Here's how the part is built. I have some questions about the finished solid (model axes, mm). A direction names the side the tool comes from. Give positions to 0.01 mm unless a question says otherwise; leave off trailing zeros. Loops run counter-clockwise (first coordinate to the right, second up) from the corner with the lowest first, then second, coordinate; pieces in that order, holes last. Notation, with made-up numbers: (58.25, 70.5) - (73.25, 70.5) arc R24 cw to (73.25, 83.5) - close; hole circle Ø4 at (-12, 83.5). An arc over 180 degrees is marked (long way). Use a Markdown table: item, result.
from build123d import *

# Parameters (mm, degrees)
SKETCH1_R           = 11.3
SKETCH1_R_2         = 4
SKETCH1_R_3         = 2
BOSS_EXTRUDE1_DEPTH = 2
FILLET1_R           = 10
SKETCH2_R           = 2.1
CUT_EXTRUDE1_DEPTH  = 182.73882359


with BuildPart() as part:
    # Sketch1 → Boss-Extrude1 (new body)
    with BuildSketch(Plane.XY):
        with BuildLine():
            ThreePointArc((0, 0), (12.5, -12.5), (25, 0))
            Line((25, 0), (25, 15))
            Line((25, 15), (17, 15))
            Line((17, 15), (17, 137.5))
            Line((17, 137.5), (25, 137.5))
            Line((25, 137.5), (25, 180))
            Line((25, 180), (0, 180))
            Line((0, 180), (0, 137.5))
            Line((0, 137.5), (8, 137.5))
            Line((8, 137.5), (8, 15))
            Line((8, 15), (0, 15))
            Line((0, 15), (0, 0))
        make_face()
        with Locations((12.5, 0)):
            Circle(SKETCH1_R, mode=Mode.SUBTRACT)
        with Locations((12.5, 150)):
            Circle(SKETCH1_R_2, mode=Mode.SUBTRACT)
        with Locations((18.156854249, 144.343145751)):
            Circle(SKETCH1_R_3, mode=Mode.SUBTRACT)
        with Locations((5.782485579, 143.282485579)):
            Circle(SKETCH1_R_3, mode=Mode.SUBTRACT)
        with Locations((19.217514421, 156.717514421)):
            Circle(SKETCH1_R_3, mode=Mode.SUBTRACT)
        with Locations((6.843145751, 155.656854249)):
            Circle(SKETCH1_R_3, mode=Mode.SUBTRACT)
    extrude(amount=BOSS_EXTRUDE1_DEPTH)

    # Fillet1
    # the kernel refuses this fillet: 10 mm, written as the material it takes off along each edge
    with BuildSketch(Plane(origin=(25, 15, -24.494897428), x_dir=(0, -1, 0), z_dir=(0, 0, 1)), Plane(origin=(0, 137.5, -24.494897428), x_dir=(0, 1, 0), z_dir=(0, 0, 1))) as fillet1_piece_1:
        with BuildLine():
            CenterArc((9.797958971, -10), FILLET1_R, 90, 78.463040967)
            Line((0, -8), (-0.195959179, -7.96))
            ThreePointArc((-0.195959179, -7.96), (-0.2, -4), (-0.2, 0))
            Line((-0.2, 0), (0, 0.2))
            Line((0, 0.2), (9.797958971, 0.2))
            Line((9.797958971, 0.2), (9.797958971, 0))
        make_face()
    extrude(amount=50.989794856, mode=Mode.SUBTRACT)
    with BuildSketch(Plane(origin=(0, 15, -24.494897428), x_dir=(1, 0, 0), z_dir=(0, 0, 1)), Plane(origin=(25, 137.5, -24.494897428), x_dir=(-1, 0, 0), z_dir=(0, 0, 1))) as fillet1_piece_2:
        with BuildLine():
            CenterArc((10, -9.797958971), FILLET1_R, 101.536959033, 78.463040967)
            Line((0, -9.797958971), (-0.2, -9.797958971))
            Line((-0.2, -9.797958971), (-0.2, 0))
            Line((-0.2, 0), (0, 0.2))
            ThreePointArc((0, 0.2), (4, 0.2), (7.96, 0.195959179))
            Line((7.96, 0.195959179), (8, 0))
        make_face()
    extrude(amount=50.989794856, mode=Mode.SUBTRACT)
    with BuildSketch(Plane(origin=(0, 180, -25), x_dir=(1, 0, 0), z_dir=(0, 0, 1)), Plane(origin=(25, 180, -25), x_dir=(0, -1, 0), z_dir=(0, 0, 1))) as fillet1_piece_3:
        with BuildLine():
            CenterArc((FILLET1_R, -FILLET1_R), FILLET1_R, 90, 90)
            Line((0, -FILLET1_R), (-FILLET1_R * 0.02, -FILLET1_R))
            Line((-FILLET1_R * 0.02, -FILLET1_R), (-FILLET1_R * 0.02, FILLET1_R * 0.02))
            Line((-FILLET1_R * 0.02, FILLET1_R * 0.02), (FILLET1_R, FILLET1_R * 0.02))
            Line((FILLET1_R, FILLET1_R * 0.02), (FILLET1_R, 0))
        make_face()
    extrude(amount=52, mode=Mode.SUBTRACT)

    # Sketch2 → Cut-Extrude1 (cut, through all)
    with BuildSketch(Plane(origin=(0, 0, 0), x_dir=(-1, 0, 0), z_dir=(0, 0, -1))):
        with Locations((-12.5, 120)):
            Circle(SKETCH2_R)
        with Locations((-12.5, 30)):
            Circle(SKETCH2_R)
        with Locations((-19.5, 170)):
            Circle(SKETCH2_R)
        with Locations(Location((-5.5, 170, 0), (0, 0, 180))):
            Circle(SKETCH2_R)
    extrude(amount=-CUT_EXTRUDE1_DEPTH, mode=Mode.SUBTRACT)


solid = part.part
(1) Suppose I cut it at A-A on y = 120. Write out the boundary of the cut face in (x, z), plus the area to 3 significant figures.
A:
| item | result |
|---|---|
| outline | (8, 0) - (10.4, 0) - (10.4, 2) - (8, 2) - close; (14.6, 0) - (17, 0) - (17, 2) - (14.6, 2) - close |
| area | 9.60 mm2 |
(2) We'd pull the mould along Y, two halves only. Please class faces 4 (the face through (22.15, 176.99, 0.99)), 5 (the face through (12.225, -12.497, 0.986)), 6 (the face through (1.21, 0.5, 0.99)): pulls with the +Y half, pulls with the -Y half, needs draft (parallel to the pull), parting line crosses it, or undercut.
A:
| item | result |
|---|---|
| face 4 | pulls with the +Y half |
| face 5 | pulls with the -Y half |
| face 6 | undercut |
(3) Suppose I cut it at C-C on y = 150. Write out the boundary of the cut face in (x, z), plus the area to 3 significant figures.
A:
| item | result |
|---|---|
| outline | (0, 0) - (8.5, 0) - (8.5, 2) - (0, 2) - close; (16.5, 0) - (25, 0) - (25, 2) - (16.5, 2) - close |
| area | 34.0 mm2 |
(4) Suppose I cut it at B-B on z = 1.45. Count the separate pieces of the cut face and the enclosed holes in it, plus the area to 3 significant figures.
A:
| item | result |
|---|---|
| separate pieces | 1 |
| enclosed holes | 10 |
| area | 2,110 mm2 |
(5) If I drill on line 1 (Y direction, x = 12.5, z = 1.15); line 2 (Y direction, x = 13.25, z = 0.4); line 3 (Y direction, x = 6.25, z = 0.9), over which ranges is the centre line in solid material (lowest first)?
A:
| item | result |
|---|---|
| line 1 | -12.5 to -11.3, 11.3 to 27.9, 32.1 to 117.9, 122.1 to 146, 154 to 180 |
| line 2 | -12.48 to -11.28, 11.28 to 28.04, 31.96 to 118.04, 121.96 to 146.07, 153.93 to 180 |
| line 3 | -10.83 to -9.41, 9.41 to 14.47, 138.03 to 141.34, 145.23 to 153.75, 157.57 to 168.04, 171.96 to 179.27 |
(6) Will these pins go through, and if not, where does the flat tip stop? pin 1 (1 mm diameter, centred on y = 59, z = 1.5, fed in from +X); pin 2 (0.6 mm diameter, centred on y = 90.5, z = 1, fed in from -X).
A:
| item | result |
|---|---|
| pin 1 | x = 17 |
| pin 2 | x = 8 |
(7) On a 3-axis mill with a long thin cutter (end or side, diameter ignored), from which of +Z, -Z, +X, -X, +Y, -Y can I reach the whole of each face in a straight line? I mean faces 1 (the face through (12.96, 117.95, 0.99)), 2 (the face through (2.19, 141.05, 0.99)), 3 (the face through (22.685, 140.899, 0.986)). Say none if no direction works.
A:
| item | result |
|---|---|
| face 1 | +Z, -Z |
| face 2 | +Z, -Z, -X |
| face 3 | +Z, -Z, +X |
